Part print with two shaded views. Sizes in mm from the minimum x, y, z corner. Coordinates: 2 decimals unless noted, no trailing zeros. Order: outer loops, then holes, each group sorted by start corner. A loop starts at its lowest first (then second) coordinate and runs counter-clockwise, first axis right, second up.
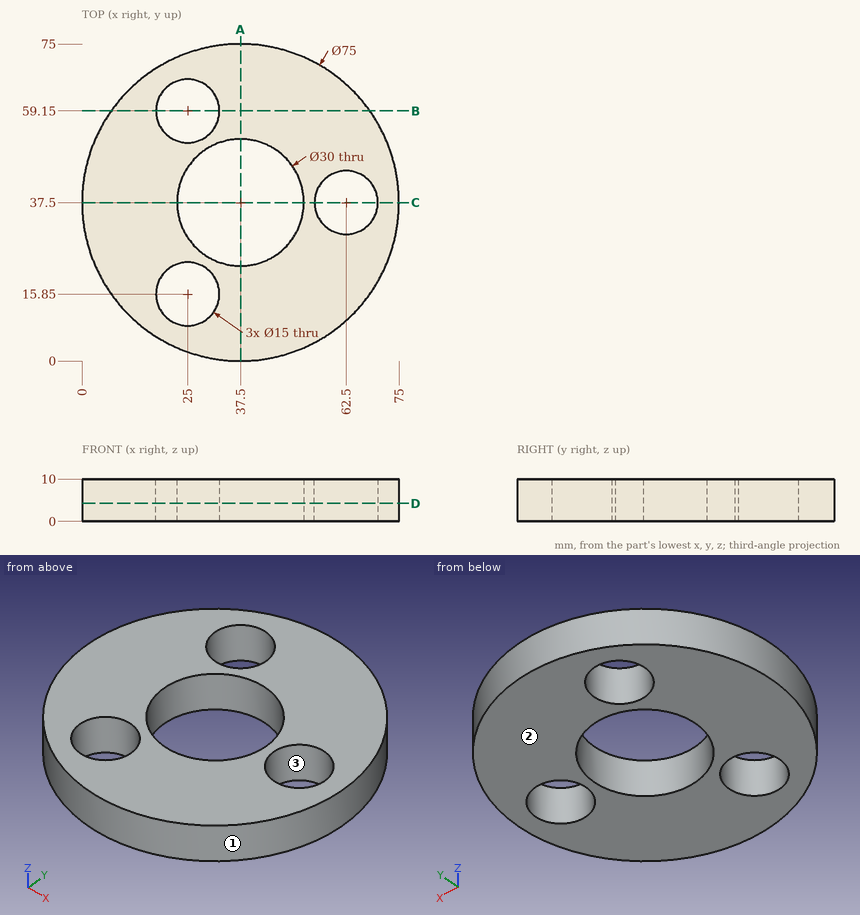
Q1. Mould opens along X. For the marked faces 1, 2 and 3 say: pulls with the +X half, pulls with the -X half, needs draft (parallel to the pull), parting line crosses it, or undercut.
Results list:
face 1: parting line crosses it
face 2: needs draft
face 3: undercut
Q2. Wall check: line 1 along Y through (x, z) = (37.5, 4.25); line 2 along Y through (x, z) = (25, 2.5); line 3 along X through (y, z) = (31.5, 1.75). Give the ranges that are in metal, low to high.
Results list:
line 1: y = 0 to 22.5, 52.5 to 75
line 2: y = 2.14 to 8.35, 23.35 to 29.21, 45.79 to 51.65, 66.65 to 72.86
line 3: x = 0.48 to 23.75, 51.25 to 58, 67 to 74.52
Q3. Cut at A-A on x = 37.5. Write the cut outline in (y, z).
Results list:
outline: (0, 0) - (22.5, 0) - (22.5, 10) - (0, 10) - close; (52.5, 0) - (75, 0) - (75, 10) - (52.5, 10) - close
Q4. Cut at D-D on z = 4.25. Write the cut outline in (x, y).
Results list:
outline: circle Ø75 at (37.5, 37.5); hole circle Ø15 at (25, 15.85); hole circle Ø15 at (25, 59.15); hole circle Ø30 at (37.5, 37.5); hole circle Ø15 at (62.5, 37.5)
Q5. Cut at B-B on y = 59.15. Write the cut outline in (x, z), and give its area (3 significant figures).
Results list:
outline: (6.88, 0) - (17.5, 0) - (17.5, 10) - (6.88, 10) - close; (32.5, 0) - (68.12, 0) - (68.12, 10) - (32.5, 10) - close
area: 462 mm2
Q6. Cut at C-C on y = 37.5. Write the cut outline in (x, z), and give its area (3 significant figures).
Results list:
outline: (0, 0) - (22.5, 0) - (22.5, 10) - (0, 10) - close; (52.5, 0) - (55, 0) - (55, 10) - (52.5, 10) - close; (70, 0) - (75, 0) - (75, 10) - (70, 10) - close
area: 300 mm2
Q7. Pin check, flat tips, straight feed: pin 1 Ø1.5 at (x, z) = (44.5, 5) entering from +Y; pin 2 Ø6 at (y, z) = (52, 6.5) entering from +X; pin 3 Ø4 at (x, z) = (36, 3) entering from -Y. Stop position of each tip, or through.
Results list:
pin 1: stops at y = 74.48
pin 2: stops at x = 73.19
pin 3: stops at y = 0
